from build123d import *

# Parameters (mm, degrees)
SKETCH1_R           = 53.975
BOSS_EXTRUDE1_DEPTH = 25.4
SKETCH2_OUTSIDE_W   = 140.902
SKETCH2_OUTSIDE_H   = 140.902
SKETCH2_OUTSIDE_R   = 41.275
CUT_EXTRUDE1_DEPTH  = 19.05
SKETCH3_R           = 28.575
CUT_EXTRUDE2_DEPTH  = 26.4
SKETCH6_R           = 32.893
SKETCH6_R_2         = 29.845
CUT_EXTRUDE3_DEPTH  = 2.032
CIRPATTERN2_COUNT   = 4
SKETCH9_R           = 2.840620424
CUT_EXTRUDE4_DEPTH  = 26.4
CIRPATTERN4_COUNT   = 6


with BuildPart() as part:
    # Sketch1 → Boss-Extrude1 (new body)
    with BuildSketch(Plane.XY):
        Circle(SKETCH1_R)
    extrude(amount=BOSS_EXTRUDE1_DEPTH)

    # Sketch2 outside → Cut-Extrude1 (cut)
    with BuildSketch(Plane.XY.offset(25.4)):
        Rectangle(SKETCH2_OUTSIDE_W, SKETCH2_OUTSIDE_H)
        Circle(SKETCH2_OUTSIDE_R, mode=Mode.SUBTRACT)
    extrude(amount=-CUT_EXTRUDE1_DEPTH, mode=Mode.SUBTRACT)

    # Sketch3 → Cut-Extrude2 (cut, through all)
    with BuildSketch(Plane.XY.offset(25.4)):
        Circle(SKETCH3_R)
    extrude(amount=-CUT_EXTRUDE2_DEPTH, mode=Mode.SUBTRACT)

    # Sketch6 → Cut-Extrude3 (cut)
    with BuildSketch(Plane.XY.offset(25.4)):
        Circle(SKETCH6_R)
        Circle(SKETCH6_R_2, mode=Mode.SUBTRACT)
    extrude(amount=-CUT_EXTRUDE3_DEPTH, mode=Mode.SUBTRACT)

    # Sketch8 → #4-40 Tapped Hole1 (revolve, cut)
    with BuildSketch(Plane(origin=(18.415, 31.895715621, 25.4), x_dir=(0, -1, 0), z_dir=(1, 0, 0))):
        Polygon((0, 0), (0, 10.966152758), (1.1303, 10.287), (1.1303, 0), align=None)
    f_4_40_tapped_hole1 = revolve(axis=Axis((18.415, 31.895715621, 31.75), (0, 0, -1)), mode=Mode.SUBTRACT)

    # CirPattern2: #4-40 Tapped Hole1 ×4 about axis
    cirpattern2_axis = Axis((0, 0, 0), (0, 0, 1))
    for i in range(1, CIRPATTERN2_COUNT):
        add(f_4_40_tapped_hole1.rotate(cirpattern2_axis, i * 360 / CIRPATTERN2_COUNT), mode=Mode.SUBTRACT)

    # Sketch9 → Cut-Extrude4 (cut, through all)
    with BuildSketch(Plane(origin=(0, 0, 0), x_dir=(-1, 0, 0), z_dir=(0, 0, -1))):
        with Locations((0, 47.625)):
            Circle(SKETCH9_R)
    cut_extrude4 = extrude(amount=-CUT_EXTRUDE4_DEPTH, mode=Mode.SUBTRACT)

    # CirPattern4: Cut-Extrude4 ×6 about axis
    cirpattern4_axis = Axis((0, 0, 0), (0, 0, 1))
    for i in range(1, CIRPATTERN4_COUNT):
        add(cut_extrude4.rotate(cirpattern4_axis, i * 360 / CIRPATTERN4_COUNT), mode=Mode.SUBTRACT)


solid = part.part
The listing builds one solid part. Answer for the finished solid, in the listing's coordinates (mm). A direction names the side the tool comes from. Round coordinates to 2 decimals unless told otherwise and drop trailing zeros. Order: outer loops, then holes, each group sorted by start corner. A loop starts at its lowest first (then second) coordinate and runs counter-clockwise, first axis right, second up. Notation, with made-up numbers: M -9.5,67.5 L 29.5,67.5 A28 cw 29.5,88.5 Z; hole C 26.25,10.5 d11. An arc over 180 degrees is marked long. Answer in a Markdown table with one row per item. Add a question column.
1) Flat-ended cylindrical pins translate along their axes: pin 1 Ø1.5 at (x, z) = (-2.5, 13) entering from +Y; pin 2 Ø9 at (x, y) = (41.24, -23.81) entering from +Z; pin 3 Ø1 at (y, z) = (-22, 4.5) entering from +X. Find the tip coordinate at first contact, or state that the pin passes through.
2) The part is cut by section D-D on y = 35. Determine the outline of the cut face in (x, z), plus the area to 3 significant figures.
3) The part is cut by section B-B on y = 0. Determine the outline of the cut face in (x, z) (3 decimals).
4) Consider line 1 along Y through (x, z) = (0, 24) (3 decimals); line 2 along X through (y, z) = (-22.5, 3); line 3 along Z through (x, y) = (-36, 26.5). Determine where each line is inside the solid, lowest interval first. Write a range as from..to.
5) The part is cut by section A-A on x = 0. Determine the outline of the cut face in (y, z) (3 decimals).
6) Which of the six approach directions +Z, -Z, +X, -X, +Y, -Y give full straight-line access (tool end or side, diameter ignored) to faces 1 (the face through (-28.547, 1.256, 12.878)), 2 (the face through (-26.103, -20.015, 24.398))?
7) The part is cut by section C-C on x = 36.5. Determine the outline of the cut face in (y, z).
8) Determine the mould class of faces 3 (the face through (-39.78, 36.48, 3.13)), 4 (the face through (-39.93, 26.33, 3.13)), 5 (the face through (-36.2, 20.2, 6.35)) for opening direction Y: pulls with the +Y half, pulls with the -Y half, needs draft (parallel to the pull), parting line crosses it, or undercut.
Findings below:
| question | item | result |
|---|---|---|
| 1 | pin 1 | stops at y = 41.24 |
| 1 | pin 2 | stops at z = 6.35 |
| 1 | pin 3 | stops at x = 49.51 |
| 2 | outline | M -41.09,0 L 41.09,0 L 41.09,6.35 L 21.88,6.35 L 21.88,25.4 L -21.88,25.4 L -21.88,6.35 L -41.09,6.35 Z |
| 2 | area | 1,360 mm² |
| 3 | outline | M -53.975,0 L -28.575,0 L -28.575,25.4 L -29.845,25.4 L -29.845,23.368 L -32.893,23.368 L -32.893,25.4 L -41.275,25.4 L -41.275,6.35 L -53.975,6.35 Z; M 28.575,0 L 53.975,0 L 53.975,6.35 L 41.275,6.35 L 41.275,25.4 L 32.893,25.4 L 32.893,23.368 L 29.845,23.368 L 29.845,25.4 L 28.575,25.4 Z |
| 4 | line 1 | y = -41.275..-32.893, -29.845..-28.575, 28.575..29.845, 32.893..41.275 |
| 4 | line 2 | x = -49.06..-43.76, -38.73..-17.61, 17.61..38.73, 43.76..49.06 |
| 4 | line 3 | z = 0..6.35 |
| 5 | outline | M -53.975,0 L -50.466,0 L -50.466,6.35 L -53.975,6.35 Z; M -44.784,0 L -28.575,0 L -28.575,25.4 L -29.845,25.4 L -29.845,23.368 L -32.893,23.368 L -32.893,25.4 L -41.275,25.4 L -41.275,6.35 L -44.784,6.35 Z; M 28.575,0 L 44.784,0 L 44.784,6.35 L 41.275,6.35 L 41.275,25.4 L 32.893,25.4 L 32.893,23.368 L 29.845,23.368 L 29.845,25.4 L 28.575,25.4 Z; M 50.466,0 L 53.975,0 L 53.975,6.35 L 50.466,6.35 Z |
| 6 | face 1 | +Z, -Z |
| 6 | face 2 | +Z |
| 7 | outline | M -39.76,0 L 39.76,0 L 39.76,6.35 L 19.27,6.35 L 19.27,25.4 L -19.27,25.4 L -19.27,6.35 L -39.76,6.35 Z |
| 8 | face 3 | parting line crosses it |
| 8 | face 4 | undercut |
| 8 | face 5 | needs draft |
